Work out the finished part from the listing and answer in its coordinate system (mm). Coordinates: 2 decimals unless noted, no trailing zeros. Write each loop counter-clockwise with the first axis right and the second up, starting at its lowest first coordinate (ties: lowest second). Pieces come first, ordered by that corner, then holes. Notation, with made-up numbers: M 73,43 L 81,43 A28 cw 81,68 Z; hole C 65.5,78.5 d8. An arc over 180 degrees is marked long. Answer as CSV lines item,"result". Start each with the question number.
(1) A cutting plane is placed at D-D on z = -30.5. Give the vertices of the cut face in (x, y) (3 decimals).
(2) A cutting plane is placed at C-C on y = -2.3. Give the vertices of the cut face in (x, z) (3 decimals), then the cut area to 3 significant figures.
(3) A cutting plane is placed at B-B on z = -13. Give the vertices of the cut face in (x, y) (3 decimals).
(4) Find the intervals of material crossed by L1, parallel to Z at x = 23, y = -2.35; L2, parallel to X at y = -2.15, z = 9 (3 decimals); L3, parallel to Z at x = 17.5, y = -1.4 (3 decimals), in increasing order. Write a range as [from, to].
(5) A cutting plane is placed at A-A on x = 14. Give the vertices of the cut face in (y, z) (3 decimals).
(6) Flat-ended cylindrical pins translate along their axes: P1, Ø1, axis at x = 43, y = -1.5, coming from the +Z side; P2, Ø1, axis at x = 25.5, y = -1, coming from the -Z side; P3, Ø1, axis at y = -2, z = 59, coming from the +X side; P4, Ø12, axis at x = -20, z = 0.5, coming from the +Y side. Find the tip coordinate at first contact, or state that the pin passes through.
from build123d import *

# Parameters (mm, degrees)
F1_DEPTH = 3.175
F2_W     = 31.75
F2_H     = 31.75
F3_DEPTH = 3.176


with BuildPart() as f1:
    # F0 (on Front) → F1 (new body)
    with BuildSketch(Plane.XZ):
        Polygon((57.15, -19.05), (60.325, -19.05), (60.325, 19.05), (57.15, 19.05), (57.15, 57.15), (19.05, 57.15), (19.05, 60.325), (-19.05, 60.325), (-19.05, 57.15), (-57.15, 57.15), (-57.15, 19.05), (-60.325, 19.05), (-60.325, 0), (-60.325, -19.05), (-57.15, -19.05), (-57.15, -57.15), (-19.05, -57.15), (-16.51, -57.15), (19.05, -57.15), (57.15, -57.15), align=None)
        Polygon((0, -60.325), (19.05, -60.325), (19.05, -57.15), (-16.51, -57.15), (-19.05, -57.15), (-19.05, -60.325), align=None)
    extrude(amount=F1_DEPTH)

    # F2 (on face) → F3 (cut, through all)
    with BuildSketch(Plane.XZ.offset(3.175)):
        with Locations((27.686, -1.651)):
            Rectangle(F2_W, F2_H)
    extrude(amount=-F3_DEPTH, mode=Mode.SUBTRACT)


solid = f1.part
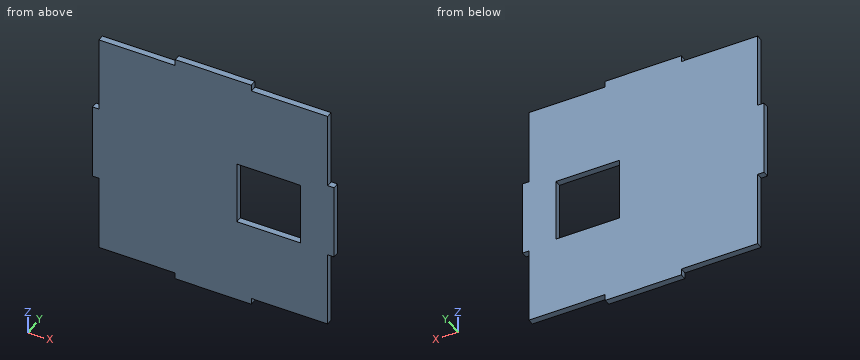
Here are the results:
1,outline,"M -57.15,-3.175 L 57.15,-3.175 L 57.15,0 L -57.15,0 Z"
2,outline,"M -60.325,-19.05 L -57.15,-19.05 L -57.15,-57.15 L -19.05,-57.15 L -19.05,-60.325 L 19.05,-60.325 L 19.05,-57.15 L 57.15,-57.15 L 57.15,-19.05 L 60.325,-19.05 L 60.325,19.05 L 57.15,19.05 L 57.15,57.15 L 19.05,57.15 L 19.05,60.325 L -19.05,60.325 L -19.05,57.15 L -57.15,57.15 L -57.15,19.05 L -60.325,19.05 Z; hole M 11.811,-17.526 L 43.561,-17.526 L 43.561,14.224 L 11.811,14.224 Z"
2,area,"12,500 mm^2"
3,outline,"M -60.325,-3.175 L 11.811,-3.175 L 11.811,0 L -60.325,0 Z; M 43.561,-3.175 L 60.325,-3.175 L 60.325,0 L 43.561,0 Z"
4,L1,"z = [-57.15, -17.53], [14.22, 57.15]"
4,L2,"x = [-60.325, 11.811], [43.561, 60.325]"
4,L3,"z = [-60.325, -17.526], [14.224, 60.325]"
5,outline,"M -3.175,-60.325 L 0,-60.325 L 0,-17.526 L -3.175,-17.526 Z; M -3.175,14.224 L 0,14.224 L 0,60.325 L -3.175,60.325 Z"
6,P1,"stops at z = 57.15"
6,P2,"stops at z = -57.15"
6,P3,"stops at x = 19.05"
6,P4,"stops at y = 0"
